from build123d import *

# Parameters (mm, degrees)
F0_W     = 120
F0_H     = 15
F1_DEPTH = 20
F2_R     = 5
F3_DEPTH = 15.001


with BuildPart() as f1:
    # F0 (on Front) → F1 (new body, symmetric)
    with BuildSketch(Plane.XZ):
        Rectangle(F0_W, F0_H)
    extrude(amount=F1_DEPTH, both=True)

    # F2 (on face) → F3 (cut, through all)
    with BuildSketch(Plane.XY.offset(7.5)):
        with Locations((-40, 0)):
            Circle(F2_R)
        with Locations((40, 0)):
            Circle(F2_R)
    extrude(amount=-F3_DEPTH, mode=Mode.SUBTRACT)


solid = f1.part
Build history of the part. All positions in model axes, mm. Give positions to 0.01 mm unless a question says otherwise; leave off trailing zeros. Order: outer loops, then holes, each group sorted by start corner. A loop starts at its lowest first (then second) coordinate and runs counter-clockwise, first axis right, second up. Notation, with made-up numbers: M -13.5,82.25 L 0.5,82.25 A26 cw 0.5,118.25 Z; hole C -33,22.25 d6. An arc over 180 degrees is marked long. Use one line per item in the form item = value.
Q1. Wall check: probe 1 along X at (y, z) = (-3, -4.75); probe 2 along Y at (x, z) = (-40, -1.5); probe 3 along X at (y, z) = (-3.5, 1.25). Give the ranges that are in metal, low to high.
Conclusion:
probe_1 = -60 to -44, -36 to 36, 44 to 60
probe_2 = -20 to -5, 5 to 20
probe_3 = -60 to -43.57, -36.43 to 36.43, 43.57 to 60
Q2. Slice it at B-B, the plane y = 0. Write the cut outline in (x, z).
Conclusion:
outline = M -60,-7.5 L -45,-7.5 L -45,7.5 L -60,7.5 Z; M -35,-7.5 L 35,-7.5 L 35,7.5 L -35,7.5 Z; M 45,-7.5 L 60,-7.5 L 60,7.5 L 45,7.5 Z
Q3. Pull direction X, two halves, no side cores. Call faces 1 (the cylindrical face through (35, 0, 0)), 2 (the flat face through (-1, 0, -7.5)), 3 (the flat face through (60, 0, 0)): released by +X, released by -X, zero draft, split by the parting line, or undercut.
Conclusion:
face_1 = undercut
face_2 = zero draft
face_3 = released by +X
Q4. Slice it at A-A, the plane x = -40. Write the cut outline in (y, z).
Conclusion:
outline = M -20,-7.5 L -5,-7.5 L -5,7.5 L -20,7.5 Z; M 5,-7.5 L 20,-7.5 L 20,7.5 L 5,7.5 Z
Q5. Slice it at C-C, the plane z = -5.5. Write the cut outline in (x, y), and give its area (3 significant figures).
Conclusion:
outline = M -60,-20 L 60,-20 L 60,20 L -60,20 Z; hole C -40,0 d10; hole C 40,0 d10
area = 4,640 mm2
